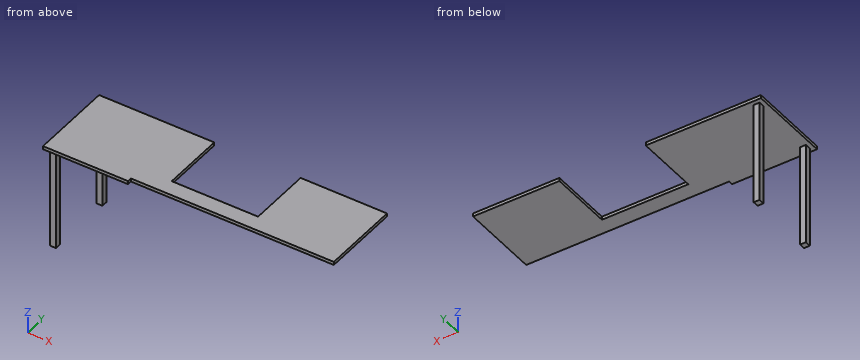
```python
from build123d import *

# Parameters (mm, degrees)
F1_DEPTH = 28.575
F2_W     = 50.8
F2_H     = 50.8
F3_DEPTH = 901.7


with BuildPart() as f1:
    # F0 (on Top) → F1 (new body)
    with BuildSketch(Plane.XY):
        Polygon((-1790.7, 0), (0, 0), (0, 698.5), (-762, 698.5), (-762, 139.7), (-1524, 139.7), (-1524, 698.5), (-2540, 698.5), (-2540, 0), (-2540, -38.1), (-1790.7, -38.1), align=None)
    extrude(amount=F1_DEPTH)

    # F2 (on face) → F3 (join)
    with BuildSketch(Plane(origin=(0, 0, 0), x_dir=(1, 0, 0), z_dir=(0, 0, -1))):
        with Locations((-2476.5, -25.4)):
            Rectangle(F2_W, F2_H)
        with Locations((-2476.5, -635)):
            Rectangle(F2_W, F2_H)
    extrude(amount=F3_DEPTH)


solid = f1.part
```
For this review, take the finished solid that the model builds, in its own axes (mm). Coordinates: 2 decimals unless noted, no trailing zeros. Write each loop counter-clockwise with the first axis right and the second up, starting at its lowest first coordinate (ties: lowest second). Pieces come first, ordered by that corner, then holes. Notation, with made-up numbers: (13.25, 32.5) - (30.25, 32.5) arc R22 cw to (30.25, 62.5) - close; hole circle Ø8 at (77, 40). An arc over 180 degrees is marked (long way). Put each result on its own line as item: value.
1. Wall thickness on probe 1 along Z at (x, y) = (-2076, 306) (3 decimals): over which ranges is the line inside the solid? List them lowest first.
Values found:
probe 1: 0 to 28.575
2. Add section D-D, the plane x = -1488. Give the boundary of the cut face in (y, z) (3 decimals), then the cut area to 3 significant figures.
Values found:
outline: (0, 0) - (139.7, 0) - (139.7, 28.575) - (0, 28.575) - close
area: 3,990 mm²
3. Add section B-B, the plane z = -543. Give the boundary of the cut face in (x, y).
Values found:
outline: (-2501.9, 0) - (-2451.1, 0) - (-2451.1, 50.8) - (-2501.9, 50.8) - close; (-2501.9, 609.6) - (-2451.1, 609.6) - (-2451.1, 660.4) - (-2501.9, 660.4) - close
4. Add section C-C, the plane x = -2291. Give the boundary of the cut face in (y, z) (3 decimals), then the cut area to 3 significant figures.
Values found:
outline: (-38.1, 0) - (698.5, 0) - (698.5, 28.575) - (-38.1, 28.575) - close
area: 21,000 mm²
5. For pin 1 (23 mm diameter, centred on x = -524, z = 7.5, fed in from -Y); pin 2 (14.5 mm diameter, centred on x = -1220.5, z = 12, fed in from +Y); pin 3 (1 mm diameter, centred on x = -441.5, y = 589.5, fed in from -Z), all flat-tipped, find the tip position at first contact; note any pin that passes through.
Values found:
pin 1: y = 0
pin 2: y = 139.7
pin 3: z = 0
6. Add section A-A, the plane y = 234. Give the boundary of the cut face in (x, z) (3 decimals), then the cut area to 3 significant figures.
Values found:
outline: (-2540, 0) - (-1524, 0) - (-1524, 28.575) - (-2540, 28.575) - close; (-762, 0) - (0, 0) - (0, 28.575) - (-762, 28.575) - close
area: 50,800 mm²
